from build123d import *

# Parameters (mm, degrees)
SKETCH1_W           = 152.4
SKETCH1_H           = 88.9
BOSS_EXTRUDE1_DEPTH = 38.1
SKETCH2_W           = 147.32
SKETCH2_H           = 83.82
CUT_EXTRUDE1_DEPTH  = 33.02
SKETCH5_W           = 10.414
SKETCH5_H           = 4.572
CUT_EXTRUDE3_DEPTH  = 2.54
FILLET1_R           = 2.54
SKETCH6_R           = 2.54
CUT_EXTRUDE4_DEPTH  = 95.194282735


with BuildPart() as part:
    # Sketch1 → Boss-Extrude1 (new body)
    with BuildSketch(Plane(origin=(0, 0, 0), x_dir=(1, 0, 0), z_dir=(0, 1, 0))):
        Rectangle(SKETCH1_W, SKETCH1_H)
    extrude(amount=BOSS_EXTRUDE1_DEPTH)

    # Sketch2 → Cut-Extrude1 (cut)
    with BuildSketch(Plane(origin=(0, 38.1, 0), x_dir=(1, 0, 0), z_dir=(0, 1, 0))):
        Rectangle(SKETCH2_W, SKETCH2_H)
    extrude(amount=-CUT_EXTRUDE1_DEPTH, mode=Mode.SUBTRACT)

    # Sketch5 → Cut-Extrude3 (cut)
    with BuildSketch(Plane.ZY.offset(76.2)):
        with Locations((0, 20.574)):
            Rectangle(SKETCH5_W, SKETCH5_H)
    extrude(amount=-CUT_EXTRUDE3_DEPTH, mode=Mode.SUBTRACT)

    # Fillet1
    fillet1_edges = [part.edges().sort_by_distance(p)[0] for p in [
        (76.2, 19.05, 44.45),
        (-76.2, 19.05, 44.45),
        (-76.2, 19.05, -44.45),
        (76.2, 19.05, -44.45),
    ]]
    fillet(fillet1_edges, radius=FILLET1_R)

    # Sketch6 → Cut-Extrude4 (cut, through all)
    with BuildSketch(Plane(origin=(0, 5.08, 0), x_dir=(1, 0, 0), z_dir=(0, 1, 0))):
        with Locations(Location((28.448, 23.114, 0), (0, 0, 270))):
            Circle(SKETCH6_R)
        with Locations(Location((28.448, -23.114, 0), (0, 0, 90))):
            Circle(SKETCH6_R)
    extrude(amount=-CUT_EXTRUDE4_DEPTH, mode=Mode.SUBTRACT)


solid = part.part
Build history of the part. All positions in model axes, mm. A direction names the side the tool comes from. Coordinates: 2 decimals unless noted, no trailing zeros. Order: outer loops, then holes, each group sorted by start corner. A loop starts at its lowest first (then second) coordinate and runs counter-clockwise, first axis right, second up. Notation, with made-up numbers: (24, -36.5) - (79, -36.5) arc R19 cw to (79, -17.5) - close; hole circle Ø5 at (74, 18). An arc over 180 degrees is marked (long way). Write item = value, one per line. Start each with the question number.
1) Saw through at A-A on y = 24.5. Write the cut outline in (x, z).
2) Wall check: line 1 along Z through (x, y) = (13.5, 22.5); line 2 along X through (y, z) = (10.5, -35); line 3 along Y through (x, z) = (51, -19). Give the ranges that are in metal, low to high. Write a range as from..to.
3) 3-axis set-ups, long thin cutter, end or side, ignore diameter. For faces 1 (the face through (-1, 22, -41.91)), 2 (the face through (30.59, 2.58, -21.75)): which of +Z, -Z, +X, -X, +Y, -Y reach the whole face in a straight line?
4) Saw through at B-B on z = 2. Write the cut outline in (x, y), then the cut area to 3 significant figures.
5) Saw through at C-C on x = 60. Write the cut outline in (y, z), then the cut area to 3 significant figures.
6) Saw through at D-D on z = -24. Write the cut outline in (x, y).
7) Two-plate mould, pull along X, no slides. Class faces 3 (the face through (-1, 5.08, -1)), 4 (the face through (76.2, 19, 1)), 5 (the face through (-73.66, 25, 1)), 6 (the face through (-1, 19, 44.45)): pulls with the +X half, pulls with the -X half, needs draft (parallel to the pull), parting line crosses it, or undercut.
8) Flat gauge pins, fed straight in: pin 1 Ø3 at (x, y) = (-75.5, 21.5) entering from -Z; pin 2 Ø8 at (x, z) = (28.448, 23.114) entering from +Y. Where does each tip first touch, or does it go through?
From the geometry:
q1.outline = (-76.2, -41.91) arc R2.54 ccw to (-73.66, -44.45) - (73.66, -44.45) arc R2.54 ccw to (76.2, -41.91) - (76.2, 41.91) arc R2.54 ccw to (73.66, 44.45) - (-73.66, 44.45) arc R2.54 ccw to (-76.2, 41.91) - close; hole (-73.66, -41.91) - (73.66, -41.91) - (73.66, 41.91) - (-73.66, 41.91) - close
q2.line_1 = -44.45..-41.91, 41.91..44.45
q2.line_2 = -76.2..-73.66, 73.66..76.2
q2.line_3 = 0..5.08
q3.face_1 = +Y
q3.face_2 = +Y, -Y
q4.outline = (-76.2, 0) - (76.2, 0) - (76.2, 38.1) - (73.66, 38.1) - (73.66, 5.08) - (-73.66, 5.08) - (-73.66, 18.29) - (-76.2, 18.29) - close; (-76.2, 22.86) - (-73.66, 22.86) - (-73.66, 38.1) - (-76.2, 38.1) - close
q4.area = 930 mm^2
q5.outline = (0, -44.45) - (38.1, -44.45) - (38.1, -41.91) - (5.08, -41.91) - (5.08, 41.91) - (38.1, 41.91) - (38.1, 44.45) - (0, 44.45) - close
q5.area = 619 mm^2
q6.outline = (-76.2, 0) - (26.07, 0) - (26.07, 5.08) - (-73.66, 5.08) - (-73.66, 38.1) - (-76.2, 38.1) - close; (30.83, 0) - (76.2, 0) - (76.2, 38.1) - (73.66, 38.1) - (73.66, 5.08) - (30.83, 5.08) - close
q7.face_3 = undercut
q7.face_4 = pulls with the +X half
q7.face_5 = undercut
q7.face_6 = needs draft
q8.pin_1 = -44.43
q8.pin_2 = 5.08
